Geometry check sheet. Reference: the model listing, model coordinates, mm. A direction names the side the tool comes from. Round coordinates to 2 decimals unless told otherwise and drop trailing zeros. Loops run counter-clockwise (first coordinate to the right, second up) from the corner with the lowest first, then second, coordinate; pieces in that order, holes last. Notation, with made-up numbers: (83, 10.5) -> (108, 10.5) arc R12 cw to (108, 18.5) -> close; hole circle Ø9 at (32.25, -36). An arc over 180 degrees is marked (long way). Use a Markdown table: item, result. Add a question column.
Q1. Sectioned sample at D-D, the plane y = -18. Enter the section's corners in (x, z).
Q2. Gauge pin test, flat ends, axial feed: P1, Ø3.5, axis at x = 1.5, y = -22.5, coming from the +Z side; P2, Ø4, axis at y = -17, z = 1.5, coming from the -X side; P3, Ø2.5, axis at x = -1.5, z = 1.5, coming from the +Y side. Record the tip position at first contact, or that the pin passes through.
Q3. Release check for a two-part mould opening along X. For faces 4 (the face through (-2, -55, 0)), 5 (the face through (-1.01, -127.12, 3.94)), 6 (the face through (-1.09, -27.53, 4.93)) record: released by +X, released by -X, zero draft, split by the parting line, or undercut.
Q4. Sectioned sample at A-A, the plane y = 0. Enter the section's corners in (x, z).
Q5. Set-up check for faces 1 (the face through (0, -13, 2)), 2 (the face through (0, -20, 4.75)), 3 (the face through (-7.5, -53, 4)): record each of +Z, -Z, +X, -X, +Y, -Y from which the full face is reachable in a straight line by a thin tool's end or side.
Q6. Material ranges on L1, parallel to X at y = -0.5, z = 0.75; L2, parallel to X at y = -100.5, z = 7.75; L3, parallel to X at y = -65.5, z = 0.75, recorded low to high.
Q7. Sectioned sample at C-C, the plane z = 6.75. Enter the section's corners in (x, y).
Q8. Sectioned sample at B-B, the plane x = 0. Enter the section's corners in (y, z).
```python
from build123d import *

# Parameters (mm, degrees)
SKETCH_R      = 30
SKETCH_R_2    = 27.55
PAD_DEPTH     = 10
POCKET_DEPTH  = 10
SKETCH002_W   = 11.2
SKETCH002_H   = 4.75
PAD001_DEPTH  = 15
SKETCH003_W   = 15
SKETCH003_H   = 8
PAD002_DEPTH  = 50
SKETCH004_R   = 25.5
SKETCH004_R_2 = 22.9
PAD003_DEPTH  = 8


with BuildPart() as body:
    # Sketch → Pad (new body)
    with BuildSketch(Plane.XY):
        Circle(SKETCH_R)
        Circle(SKETCH_R_2, mode=Mode.SUBTRACT)
    extrude(amount=PAD_DEPTH)

    # Sketch001 (on Face4 of Pad) → Pocket (cut)
    with BuildSketch(Plane.XY.offset(10)):
        with BuildLine():
            ThreePointArc((33.724741, 20.89253), (0.382596, 39.670008), (-33.31551, 21.539098))
            Line((-33.31551, 21.539098), (0, 0))
            Line((0, 0), (33.724741, 20.89253))
        make_face()
    extrude(amount=-POCKET_DEPTH, mode=Mode.SUBTRACT)


with BuildPart() as fusion:
    # Sketch002 → Pad001 (new body)
    with BuildSketch(Plane.XZ.offset(20)):
        with Locations((0, 2.375)):
            Rectangle(SKETCH002_W, SKETCH002_H)
    extrude(amount=PAD001_DEPTH)


with BuildPart() as fusion_1:
    # Body001 placement: moved
    add(fusion.part.moved(Location((0, 7, 0))))

    # Fusion: union Body
    add(body.part)


with BuildPart() as fusion001:
    # Sketch003 (on Body) → Pad002 (new body)
    with BuildSketch(Plane.XZ.offset(-7)):
        with Locations((0, 4)):
            Rectangle(SKETCH003_W, SKETCH003_H)
    extrude(amount=PAD002_DEPTH)


with BuildPart() as fusion001_1:
    # Body002 placement: moved
    add(fusion001.part.moved(Location((0, -35.2, 0))))

    # Fusion001: union Fusion
    add(fusion_1.part)


with BuildPart() as fusion002:
    # Sketch004 → Pad003 (new body)
    with BuildSketch(Plane.XY):
        with Locations((0, -84.238922)):
            Circle(SKETCH004_R)
        with Locations((0, -84.238922)):
            Circle(SKETCH004_R_2, mode=Mode.SUBTRACT)
    extrude(amount=PAD003_DEPTH)


with BuildPart() as fusion002_1:
    # Body003 placement: moved
    add(fusion002.part.moved(Location((0, -17.4, 0))))

    # Fusion002: union Fusion001
    add(fusion001_1.part)


solid = fusion002_1.part
```
Values:
| question | item | result |
|---|---|---|
| 1 | outline | (-24, 0) -> (-20.86, 0) -> (-20.86, 10) -> (-24, 10) -> close; (-5.6, 0) -> (5.6, 0) -> (5.6, 4.75) -> (-5.6, 4.75) -> close; (20.86, 0) -> (24, 0) -> (24, 10) -> (20.86, 10) -> close |
| 2 | P1 | z = 4.75 |
| 2 | P2 | x = -25.98 |
| 2 | P3 | y = -13 |
| 3 | face 4 | zero draft |
| 3 | face 5 | split by the parting line |
| 3 | face 6 | undercut |
| 4 | outline | (-30, 0) -> (-27.55, 0) -> (-27.55, 10) -> (-30, 10) -> close; (27.55, 0) -> (30, 0) -> (30, 10) -> (27.55, 10) -> close |
| 5 | face 1 | +Z, -Z, +Y |
| 5 | face 2 | +Z, +Y |
| 5 | face 3 | +Z, -Z, -X |
| 6 | L1 | -30 to -27.55, 27.55 to 30 |
| 6 | L2 | -25.47 to -22.87, 22.87 to 25.47 |
| 6 | L3 | -7.5 to 7.5 |
| 7 | outline | (-25.19, 16.29) arc R30 ccw to (-7.5, -29.05) -> (-7.5, -77.27) arc R25.5 ccw (long way) to (7.5, -77.27) -> (7.5, -29.05) arc R30 ccw to (25.5, 15.8) -> (23.42, 14.51) arc R27.55 cw (long way) to (-23.14, 14.96) -> close; hole circle Ø45.8 at (0, -101.64) |
| 8 | outline | (-127.14, 0) -> (-124.54, 0) -> (-124.54, 8) -> (-127.14, 8) -> close; (-78.74, 0) -> (-13, 0) -> (-13, 4.75) -> (-27.55, 4.75) -> (-27.55, 10) -> (-30, 10) -> (-30, 8) -> (-78.74, 8) -> close |
